The listing builds one solid part. Answer for the finished solid, in the listing's coordinates (mm). A direction names the side the tool comes from. Round coordinates to 2 decimals unless told otherwise and drop trailing zeros. Order: outer loops, then holes, each group sorted by start corner. A loop starts at its lowest first (then second) coordinate and runs counter-clockwise, first axis right, second up. Notation, with made-up numbers: (-6.5, 17) -> (35.5, 17) arc R20 ccw to (35.5, 24) -> close; hole circle Ø9 at (85, 79.5). An arc over 180 degrees is marked (long way). Answer in a Markdown table with one row per item. Add a question column.
```python
from build123d import *

# Parameters (mm, degrees)
BOSS_EXTRUDE1_DEPTH = 32
FILLET1_R           = 16
SKETCH4_R           = 10
BOSS_EXTRUDE4_DEPTH = 5


with BuildPart() as part:
    # Sketch1 → Boss-Extrude1 (new body)
    with BuildSketch(Plane.XY):
        Polygon((0, 0), (0, 46), (42.2, 46), (42.2, 0), (40, 0), (40, 43.8), (2.2, 43.8), (2.2, 0), align=None)
    extrude(amount=BOSS_EXTRUDE1_DEPTH)

    # Fillet1
    fillet1_edges = [part.edges().sort_by_distance(p)[0] for p in [
        (41.1, 0, 32),
        (41.1, 0, 0),
        (1.1, 0, 0),
        (1.1, 0, 32),
    ]]
    fillet(fillet1_edges, radius=FILLET1_R - 0.0001)  # a hair under: the kernel refuses the full size

    # Sketch4 → Boss-Extrude4 (add)
    with BuildSketch(Plane(origin=(2.2, 0, 0), x_dir=(0, 0, -1), z_dir=(1, 0, 0))):
        with Locations(Location((-16, 16, 0), (0, 0, 270))):
            Circle(SKETCH4_R)
    boss_extrude4 = extrude(amount=BOSS_EXTRUDE4_DEPTH)

    # Mirror1: Boss-Extrude4 across plane
    add(boss_extrude4.mirror(Plane(origin=(21.1, 0, 0), x_dir=(0, 0, 1), z_dir=(1, 0, 0))))


solid = part.part
```
Item 1: The part is cut by section B-B, the plane z = 20. Give the vertices of the cut face in (x, y).
Item 2: For a pull along Y with two mould halves and no side action, classify faces 5 (the face through (1.085, 4.563, 4.811)), 6 (the face through (2.2, 27, 16)), 7 (the face through (0, 23, 16)), 8 (the face through (21, 46, 16)) as released by +Y, released by -Y, zero draft, split by the parting line, or undercut.
Item 3: Find the intervals of material crossed by probe 1 along X at (y, z) = (25, 9); probe 2 along X at (y, z) = (14, 7.5); probe 3 along Y at (x, z) = (20, 9), in increasing order. Write a range as [from, to].
Item 4: Flat-ended cylindrical pins translate along their axes: P1, Ø6, axis at y = 13.5, z = 13, coming from the -X side; P2, Ø6, axis at x = 33.5, y = 20.5, coming from the -Z side; P3, Ø12, axis at x = 6, z = 24, coming from the -Y side; P4, Ø4, axis at x = 32.5, y = 27, coming from the -Z side. Find the tip coordinate at first contact, or state that the pin passes through.
Item 5: The part is cut by section C-C, the plane x = 22.5. Give the vertices of the cut face in (y, z).
Item 6: A tool of negligible diameter and unlimited length cuts with its end or side. For faces 1 (the face through (21, 43.8, 16)), 2 (the face through (37.53, 6.46, 13)), 3 (the face through (41.085, 4.563, 27.189)), 4 (the face through (7.2, 16, 16)), from which of +Z, -Z, +X, -X, +Y, -Y can it reach the whole face along a straight path? Write none if from no direction.
Item 7: The part is cut by section A-A, the plane y = 12. Give the vertices of the cut face in (x, z).
Item 8: The part is cut by section D-D, the plane z = 3.5. Give the vertices of the cut face in (x, y).
Resolved:
| question | item | result |
|---|---|---|
| 1 | outline | (0, 0.51) -> (2.2, 0.51) -> (2.2, 6.83) -> (7.2, 6.83) -> (7.2, 25.17) -> (2.2, 25.17) -> (2.2, 43.8) -> (40, 43.8) -> (40, 25.17) -> (35, 25.17) -> (35, 6.83) -> (40, 6.83) -> (40, 0.51) -> (42.2, 0.51) -> (42.2, 46) -> (0, 46) -> close |
| 2 | face 5 | released by -Y |
| 2 | face 6 | undercut |
| 2 | face 7 | zero draft |
| 2 | face 8 | released by +Y |
| 3 | probe 1 | [0, 2.2], [40, 42.2] |
| 3 | probe 2 | [0, 7.2], [35, 42.2] |
| 3 | probe 3 | [43.8, 46] |
| 4 | P1 | x = 0 |
| 4 | P2 | z = 6.18 |
| 4 | P3 | y = 0.36 |
| 4 | P4 | through |
| 5 | outline | (43.8, 0) -> (46, 0) -> (46, 32) -> (43.8, 32) -> close |
| 6 | face 1 | +Z, -Z |
| 6 | face 2 | none |
| 6 | face 3 | +Z, +X, -X, -Y |
| 6 | face 4 | +Z, -Z, -Y |
| 7 | outline | (0, 0.51) -> (2.2, 0.51) -> (2.2, 6.83) -> (7.2, 6.83) -> (7.2, 25.17) -> (2.2, 25.17) -> (2.2, 31.49) -> (0, 31.49) -> close; (35, 6.83) -> (40, 6.83) -> (40, 0.51) -> (42.2, 0.51) -> (42.2, 31.49) -> (40, 31.49) -> (40, 25.17) -> (35, 25.17) -> close |
| 8 | outline | (0, 6.01) -> (2.2, 6.01) -> (2.2, 43.8) -> (40, 43.8) -> (40, 6.01) -> (42.2, 6.01) -> (42.2, 46) -> (0, 46) -> close |
